from build123d import *

# Parameters (mm, degrees)
F0_R          = 254
F1_DEPTH      = 508
F2_W          = 50.8
F2_H          = 50.8
F3_DEPTH      = 25.4
F3_DEPTH_BACK = 1134


# Not quite as in the source:
# - an extrude ends at something that could not be found from the text; its depth is read off the source's solid


with BuildPart() as f1:
    # F0 (on Front) → F1 (new body)
    with BuildSketch(Plane.XZ):
        with Locations((0, 1.6020847252)):
            Circle(F0_R)
    extrude(amount=F1_DEPTH)

    # F2 (on face) → F3 (cut, two sides)
    with BuildSketch(Plane.XZ.offset(508)) as f3_sk:
        with Locations((24.2332161129, -14.1495072007)):
            Rectangle(F2_W, F2_H)
    extrude(amount=-F3_DEPTH, mode=Mode.SUBTRACT)
    extrude(f3_sk.sketch, amount=F3_DEPTH_BACK, mode=Mode.SUBTRACT)


solid = f1.part
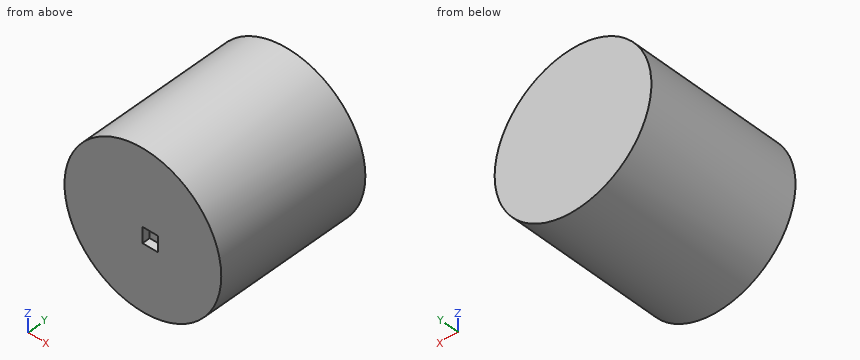
Read the model definition and answer for the solid it produces. Units are mm, in the model's axes. Coordinates: 2 decimals unless noted, no trailing zeros. Loops run counter-clockwise (first coordinate to the right, second up) from the corner with the lowest first, then second, coordinate; pieces in that order, holes last. Notation, with made-up numbers: (46.25, 10.25) -> (93.25, 10.25) arc R10 cw to (93.25, 15.25) -> close; hole circle Ø7 at (-24.5, 37). An arc over 180 degrees is marked (long way). Answer in a Markdown table with one row per item.
Item 1: A cutting plane is placed at B-B on z = -214. Determine the outline of the cut face in (x, y).
Returned:
| item | result |
|---|---|
| outline | (-134.28, -508) -> (134.28, -508) -> (134.28, 0) -> (-134.28, 0) -> close |
Item 2: A cutting plane is placed at C-C on y = -226. Determine the outline of the cut face in (x, z), plus the area to 3 significant figures.
Returned:
| item | result |
|---|---|
| outline | circle Ø508 at (0, 1.6) |
| area | 203,000 mm^2 |
Item 3: A cutting plane is placed at A-A on x = -134. Determine the outline of the cut face in (y, z).
Returned:
| item | result |
|---|---|
| outline | (-508, -214.18) -> (0, -214.18) -> (0, 217.38) -> (-508, 217.38) -> close |
Item 4: Each of these flat-tipped pins is pushed along its axis until it touches: P1, Ø12.5, axis at y = -499, z = -25.5, coming from the -X side; P2, Ø4, axis at x = 159.5, y = -346, coming from the +Z side; P3, Ø15, axis at x = 25.5, z = -9, coming from the -Y side; P4, Ø8, axis at x = -110, z = -49, coming from the +Y side. Where does it stop, or does it pass through?
Returned:
| item | result |
|---|---|
| P1 | stops at x = -253.14 |
| P2 | stops at z = 200.88 |
| P3 | stops at y = -482.6 |
| P4 | stops at y = 0 |
Item 5: Straight lines are drawn through the part: line 1 along Z through (x, y) = (-5.5, -469); line 2 along X through (y, z) = (-463, 199); line 3 along Z through (x, y) = (203, -107). For each, find the intervals that lie inside material, in ascending order. Write a range as [from, to].
Returned:
| item | result |
|---|---|
| line 1 | z = [-252.34, 255.54] |
| line 2 | x = [-159.84, 159.84] |
| line 3 | z = [-151.06, 154.27] |
